from build123d import *

# Parameters (mm, degrees)
RESSALTO_EXTRUS_O1_DEPTH = 1.5
ESBO_O2_R                = 2
RESSALTO_EXTRUS_O2_DEPTH = 7
CORTE_EXTRUS_O1_REACH    = 17.604
ESBO_O3_R                = 0.85


with BuildPart() as part:
    # Esboço1 → Ressalto-extrusão1 (new, symmetric)
    with BuildSketch(Plane.XY):
        with BuildLine():
            Line((0, 3.5), (10, 3.5))
            ThreePointArc((10, 3.5), (13.5, 0), (10, -3.5))
            Line((10, -3.5), (0, -3.5))
            ThreePointArc((0, -3.5), (-3.5, 0), (0, 3.5))
        make_face()
    extrude(amount=RESSALTO_EXTRUS_O1_DEPTH, both=True)

    # Esboço2 → Ressalto-extrusão2 (add)
    with BuildSketch(Plane(origin=(0, 0, -1.5), x_dir=(-1, 0, 0), z_dir=(0, 0, -1))):
        with Locations(Location((-10, 0, 0), (0, 0, 180))):
            Circle(ESBO_O2_R)
    extrude(amount=RESSALTO_EXTRUS_O2_DEPTH)

    # Esboço3 → Corte-extrusão1 (cut, up to next)
    with BuildSketch(Plane(origin=(0, 0, -1.5), x_dir=(-1, 0, 0), z_dir=(0, 0, -1)), mode=Mode.PRIVATE) as corte_extrus_o1_sk1:
        Circle(ESBO_O3_R)
    corte_extrus_o1_tool1 = extrude(corte_extrus_o1_sk1.sketch, amount=-CORTE_EXTRUS_O1_REACH, mode=Mode.PRIVATE) & part.part
    add(corte_extrus_o1_tool1.solids().sort_by_distance((0, 0, -1.5))[0], mode=Mode.SUBTRACT)


solid = part.part
Part model, mm, in its own coordinate system. A direction names the side the tool comes from. Coordinates: 2 decimals unless noted, no trailing zeros. Order: outer loops, then holes, each group sorted by start corner. A loop starts at its lowest first (then second) coordinate and runs counter-clockwise, first axis right, second up.
(1) Slice it at B-B, the plane z = -1.25. Write the cut outline in (x, y), and give its area (3 significant figures).
Check sheet entries:
outline: (0, -3.5) - (10, -3.5) arc R3.5 ccw to (10, 3.5) - (0, 3.5) arc R3.5 ccw to start; hole circle Ø1.7 at (0, 0)
area: 106 mm2
(2) Slice it at D-D, the plane x = 11.25. Write the cut outline in (y, z).
Check sheet entries:
outline: (-3.27, -1.5) - (-1.56, -1.5) - (-1.56, -8.5) - (1.56, -8.5) - (1.56, -1.5) - (3.27, -1.5) - (3.27, 1.5) - (-3.27, 1.5) - close
(3) Slice it at A-A, the plane y = 0. Write the cut outline in (x, z).
Check sheet entries:
outline: (-3.5, -1.5) - (-0.85, -1.5) - (-0.85, 1.5) - (-3.5, 1.5) - close; (0.85, -1.5) - (8, -1.5) - (8, -8.5) - (12, -8.5) - (12, -1.5) - (13.5, -1.5) - (13.5, 1.5) - (0.85, 1.5) - close
(4) Tool access for faces 1 (the face through (8.4, 1.2, -5)), 2 (the face through (5, 0, 1.5)): list every direction of +Z, -Z, +X, -X, +Y, -Y with a clear straight run to the whole face (end or side of a thin tool).
Check sheet entries:
face 1: -Z
face 2: +Z, +X, -X, +Y, -Y
(5) Pull direction Y, two halves, no side cores. Call faces 3 (the face through (0.18, -0.83, -0.02)), 4 (the face through (5, 0, -1.5)), 5 (the face through (5, 3.5, 0)): pulls with the +Y half, pulls with the -Y half, needs draft (parallel to the pull), parting line crosses it, or undercut.
Check sheet entries:
face 3: undercut
face 4: needs draft
face 5: pulls with the +Y half
(6) Probe L1, parallel to Y at x = 0, z = -0.3; L2, parallel to Z at x = 5.5, y = -2; L3, parallel to X at y = 1, z = -8. List the from-to ranges inside material, lowest first.
Check sheet entries:
L1: y = -3.5 to -0.85, 0.85 to 3.5
L2: z = -1.5 to 1.5
L3: x = 8.27 to 11.73
(7) Pin check, flat tip, straight feed: pin 1 Ø3 at (x, z) = (8.5, -5.5) entering from +Y. Stop position of the tip, or through.
Check sheet entries:
pin 1: stops at y = 2
(8) Slice it at C-C, the plane z = -5.75. Write the cut outline in (x, y), and give its area (3 significant figures).
Check sheet entries:
outline: circle Ø4 at (10, 0)
area: 12.6 mm2
